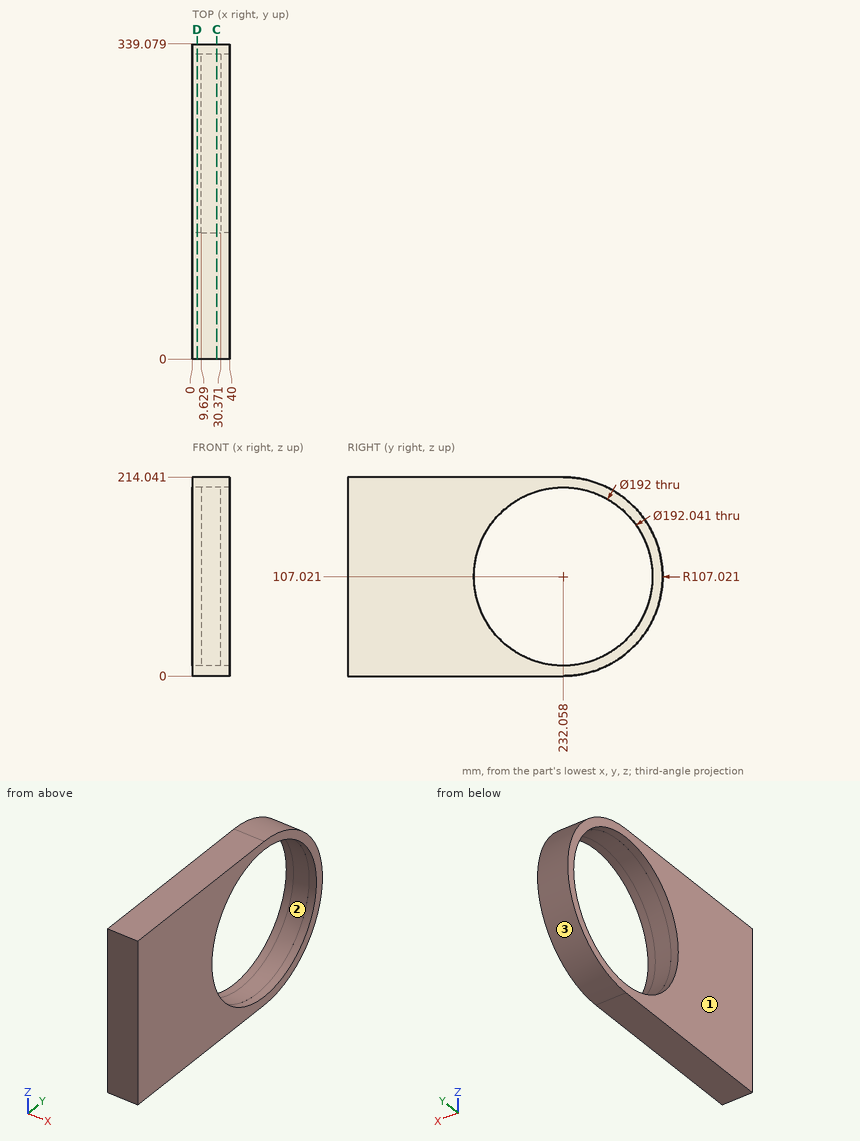
The figure shows three views and two pictorial views of one solid part (mm, origin at its lowest corner). Answer the questions. Give positions to 0.01 mm unless a question says otherwise; leave off trailing zeros. Write each loop counter-clockwise with the first axis right and the second up, starting at its lowest first coordinate (ties: lowest second). Pieces come first, ordered by that corner, then holes. Notation, with made-up numbers: M -34,-12 L -7,-12 A31 cw -7,23 Z; hole C 86,-36 d10. An arc over 180 degrees is marked long. Write each question's results on one line, items separated by ' | '.
Q1. Flat-ended cylindrical pins translate along their axes: P1, Ø5, axis at x = 12, y = 266, coming from the -Z side; P2, Ø2, axis at x = 10, z = 161.5, coming from the +Y side. Find the tip coordinate at first contact, or state that the pin passes through.
Output values:
P1: z = 4.72 | P2: y = 324.76
Q2. For a pull along Y with two mould halves and no side action, classify the marked faces 1, 2 and 3 as released by +Y, released by -Y, zero draft, split by the parting line, or undercut.
Output values:
face 1: zero draft | face 2: undercut | face 3: released by +Y
Q3. Section C-C, the plane x = 26 is taken. Write down the section's boundary in (y, z), then the cut area to 3 significant figures.
Output values:
outline: M 0,0 L 232.06,0 A107.02 ccw 232.06,214.04 L 0,214.04 Z; hole C 232.06,107.02 d192 | area: 38,700 mm2
Q4. Consider L1, parallel to Z at x = 22, y = 229.5 (1 decimal); L2, parallel to Y at x = 37.5, z = 190 (1 decimal); L3, parallel to Y at x = 3, z = 181.5 (1 decimal). Determine where each line is inside the solid, lowest interval first. Write a range as from..to.
Output values:
L1: 0..11.1, 203..214 | L2: 0..183.7, 280.4..299.6 | L3: 0..171.5, 292.7..308.9
Q5. Section D-D, the plane x = 5 is taken. Write down the section's boundary in (y, z), then the cut area to 3 significant figures.
Output values:
outline: M 0,0 L 232.06,0 A107.02 ccw 232.06,214.04 L 0,214.04 Z; hole C 232.06,107.02 d192.04 | area: 38,700 mm2
